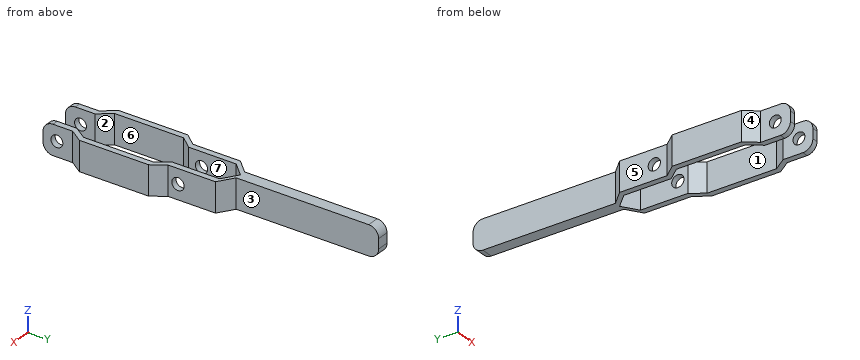
from build123d import *

# Parameters (mm, degrees)
F1_DEPTH = 15
F2_R     = 5
F3_R     = 5
F4_R     = 3.105154
F5_DEPTH = 25
F6_R     = 3
F7_DEPTH = 25


with BuildPart() as f1:
    # F0 (on Top) → F1 (new body)
    with BuildSketch(Plane.XY):
        Polygon((3, 72), (-3, 72), (-3, 0), (-9.367348, -6.612246), (-9.367348, -30.612246), (-14.458097, -36.783492), (-14.458097, -71.783492), (-9.532944, -78.087687), (-9.532944, -93.087687), (-6.532944, -93.087687), (-6.532944, -78.087687), (-11.458097, -71.783492), (-11.458097, -36.783492), (-6.367348, -30.612246), (-6.367348, -6.612246), (0, 0), (7.561686, -5.204405), (7.561686, -29.204405), (11.999285, -35.860809), (11.999285, -70.860809), (7.467056, -77.453145), (7.467056, -92.453145), (10.467056, -92.453145), (10.467056, -77.453145), (14.999285, -70.860809), (14.999285, -35.860809), (10.561686, -29.204405), (10.561686, -5.204405), (3, 0), align=None)
    extrude(amount=F1_DEPTH)

    # F2
    f2_edges = [f1.edges().sort_by_distance(p)[0] for p in [
        (-8.032944, -93.087687, 15),
        (-8.032944, -93.087687, 0),
        (8.967056, -92.453145, 15),
        (8.967056, -92.453145, 0),
    ]]
    fillet(f2_edges, radius=F2_R)

    # F3
    f3_edges = [f1.edges().sort_by_distance(p)[0] for p in [
        (0, 72, 15),
        (0, 72, 0),
    ]]
    fillet(f3_edges, radius=F3_R)

    # F4 (on face) → F5 (cut)
    with BuildSketch(Plane.YZ.offset(10.561686)):
        with Locations((-24.143221, 7.553654)):
            Circle(F4_R)
    extrude(amount=-F5_DEPTH, mode=Mode.SUBTRACT)

    # F6 (on face) → F7 (cut)
    with BuildSketch(Plane.YZ.offset(10.467056)):
        with Locations((-85.437857, 7.5)):
            Circle(F6_R)
    extrude(amount=-F7_DEPTH, mode=Mode.SUBTRACT)


solid = f1.part
Design review of the part built by this model. Coordinates are the model's own, in mm. Face numbers are marked on the shaded views. A direction names the side the tool comes from. Round coordinates to 2 decimals unless told otherwise and drop trailing zeros. Write each loop counter-clockwise with the first axis right and the second up, starting at its lowest first coordinate (ties: lowest second). Pieces come first, ordered by that corner, then holes. Notation, with made-up numbers: (84, -20) - (89, -20) arc R13 ccw to (89, 4) - close; hole circle Ø10 at (50, 57.25). An arc over 180 degrees is marked (long way). Use a Markdown table: item, result. Add a question column.
1. We need section C-C (x = 4.75). State the section outline as (y, z) points, then the cut area to 3 significant figures.
2. Mouldability with a two-part tool opening along Y and no side actions: class the marked faces 1, 2, 3 and 4 as +Y half, -Y half, draft (parallel to the pull), parting line (faces both ways), or undercut.
3. Wall thickness on probe 1 along X at (y, z) = (-23, 12.5); probe 2 along X at (y, z) = (-80.5, 8.5); probe 3 along Y at (x, z) = (-8.5, 5.5): over which ranges is each line inside the solid? List them lowest first.
4. We need section B-B (y = 10). State the section outline as (x, z) points.
5. Clearance check with flat-ended pins moving along their axes: pin 1 (7.5 mm diameter, centred on y = -19, z = 6.5, fed in from +X); pin 2 (6 mm diameter, centred on x = 11.5, z = 6, fed in from +Y); pin 3 (6 mm diameter, centred on x = -9.5, z = 5, fed in from +Y); pin 4 (3 mm diameter, centred on x = -9.5, z = 11, fed in from -Y). State where each tip first meets the part, or that it passes through.
6. For the marked faces 5, 6 and 7, list the 3-axis set-ups (+Z, -Z, +X, -X, +Y, -Y) from which the entire face can be reached by the end or side of a thin tool; tool diameter is ignored.
7. We need section A-A (y = -47). State the section outline as (x, z) points, then the cut area to 3 significant figures.
Output:
| question | item | result |
|---|---|---|
| 1 | outline | (-3.27, 0) - (-1.2, 0) - (-1.2, 15) - (-3.27, 15) - close |
| 1 | area | 31.0 mm2 |
| 2 | face 1 | undercut |
| 2 | face 2 | undercut |
| 2 | face 3 | draft |
| 2 | face 4 | -Y half |
| 3 | probe 1 | x = -9.37 to -6.37, 7.56 to 10.56 |
| 3 | probe 2 | x = -9.53 to -6.53, 7.47 to 10.47 |
| 3 | probe 3 | y = -93.09 to -87.67, -83.2 to -75.57, -33.2 to -26.47, -21.81 to -5.71 |
| 4 | outline | (-3, 0) - (3, 0) - (3, 15) - (-3, 15) - close |
| 5 | pin 1 | stops at x = 10.56 |
| 5 | pin 2 | stops at y = -3.79 |
| 5 | pin 3 | stops at y = -3.63 |
| 5 | pin 4 | stops at y = -93.09 |
| 6 | face 5 | +Z, -Z, -X, +Y |
| 6 | face 6 | +Z, -Z |
| 6 | face 7 | +Z, -Z, -Y |
| 7 | outline | (-14.46, 0) - (-11.46, 0) - (-11.46, 15) - (-14.46, 15) - close; (12, 0) - (15, 0) - (15, 15) - (12, 15) - close |
| 7 | area | 90.0 mm2 |
